```python
from build123d import *

# Parameters (mm, degrees)
F2_R      = 1.5
F3_DEPTH  = 5
F5_D      = 5.25
F5_DEPTH  = 7
F5_TIP    = 1.5772591249
F7_R      = 5
F8_DEPTH  = 2
F10_D     = 5.25
F10_DEPTH = 6.25
F10_TIP   = 1.5772591249
F12_R     = 5
F13_DEPTH = 2
F15_D     = 5.25
F15_DEPTH = 6.25
F15_TIP   = 1.5772591249
F16_R     = 12.5
F17_DEPTH = 9.5
F18_SIZE  = 2.5
F20_DEPTH = 17


with BuildPart() as f1:
    # F0 (on Front) → F1 (revolve)
    with BuildSketch(Plane.XZ):
        Polygon((0, 0), (0, 5), (0, 15.5), (-18, 15.5), (-18, 7), (-20, 7), (-20, 5), (-20, 0), align=None)
    revolve(axis=Axis((-5.3004380733, 0, 0), (-1, 0, 0)))

    # F2 (on face) → F3 (cut)
    with BuildSketch(Plane(origin=(-18, 0, 0), x_dir=(0, -1, 0), z_dir=(-1, 0, 0))):
        with Locations((8.25, 8.25)):
            Circle(F2_R)
        with Locations((-8.25, 8.25)):
            Circle(F2_R)
        with Locations((-8.25, -8.25)):
            Circle(F2_R)
        with Locations((8.25, -8.25)):
            Circle(F2_R)
    extrude(amount=-F3_DEPTH, mode=Mode.SUBTRACT)

    # F5
    with Locations(Plane(origin=(-18, 0, 0), x_dir=(0, -1, 0), z_dir=(-1, 0, 0))):
        with Locations((-8.25, 8.25), (8.25, 8.25), (-8.25, -8.25), (8.25, -8.25)):
            Hole(F5_D / 2, depth=F5_DEPTH)
            with Locations((0, 0, -(F5_DEPTH + F5_TIP / 2))):  # 118° drill point
                Cone(0, F5_D / 2, F5_TIP, mode=Mode.SUBTRACT)

    # F7 (on offset) → F8 (cut)
    with BuildSketch(Plane.XZ.offset(15.5)):
        with Locations((-7, 0)):
            Circle(F7_R)
    extrude(amount=-F8_DEPTH, mode=Mode.SUBTRACT)

    # F10
    with Locations(Plane.XZ.offset(13.5)):
        with Locations((-7, 0)):
            Hole(F10_D / 2, depth=F10_DEPTH)
            with Locations((0, 0, -(F10_DEPTH + F10_TIP / 2))):  # 118° drill point
                Cone(0, F10_D / 2, F10_TIP, mode=Mode.SUBTRACT)

    # F12 (on offset) → F13 (cut)
    with BuildSketch(Plane.XZ.offset(-15.5)):
        with Locations((-8, 0)):
            Circle(F12_R)
    extrude(amount=F13_DEPTH, mode=Mode.SUBTRACT)

    # F15
    with Locations(Plane(origin=(0, 13.5, 0), x_dir=(-1, 0, 0), z_dir=(0, 1, 0))):
        with Locations((8, 0)):
            Hole(F15_D / 2, depth=F15_DEPTH)
            with Locations((0, 0, -(F15_DEPTH + F15_TIP / 2))):  # 118° drill point
                Cone(0, F15_D / 2, F15_TIP, mode=Mode.SUBTRACT)

    # F16 (on face) → F17 (join)
    with BuildSketch(Plane.YZ):
        Circle(F16_R)
    extrude(amount=F17_DEPTH)

    # F18
    f18_edges = [f1.edges().sort_by_distance(p)[0] for p in [
        (9.5, -12.5, 0),
    ]]
    chamfer(f18_edges, length=F18_SIZE)

    # F19 (on face) → F20 (cut)
    with BuildSketch(Plane(origin=(-18, 0, 0), x_dir=(0, -1, 0), z_dir=(-1, 0, 0))):
        with BuildLine():
            Line((-14.6714007511, -5), (-14.6714007511, 5))
            ThreePointArc((-14.6714007511, 5), (-15.5, 0), (-14.6714007511, -5))
        make_face()
        with BuildLine():
            ThreePointArc((14.6714007511, -5), (15.5, 0), (14.6714007511, 5))
            Line((14.6714007511, 5), (14.6714007511, -5))
        make_face()
    extrude(amount=-F20_DEPTH, mode=Mode.SUBTRACT)


solid = f1.part
```
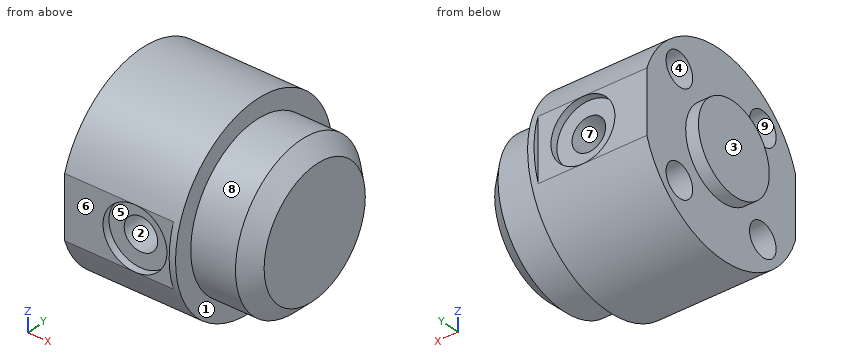
For this review, take the finished solid that the model builds, in its own axes (mm). Face numbers are marked on the shaded views. A direction names the side the tool comes from. Round coordinates to 2 decimals unless told otherwise and drop trailing zeros. Write each loop counter-clockwise with the first axis right and the second up, starting at its lowest first coordinate (ties: lowest second). Pieces come first, ordered by that corner, then holes. Notation, with made-up numbers: (-13, -36) -> (23, -36) arc R20 cw to (23, -21) -> close; hole circle Ø8 at (40, 2). An arc over 180 degrees is marked (long way). One line per question, with ' | ' between items. Start each with the question number.
1) Add section B-B (y = -13). Write out the cut boundary in (x, z) (3 decimals), and give its area (3 significant figures).
2) Wall thickness on line 1 along X through (y, z) = (14.4, 0); line 2 along Z through (x, y) = (-15.5, 8.25) (3 decimals): over which ranges is each line inside the solid? List them lowest first.
3) Machinability: for the marked faces 5, 6, 7, 8 and 9, which of the approach directions +Z, -Z, +X, -X, +Y, -Y give a long, thin tool a straight path to every point of the face, cutting with its end or side? Answer none if there is none.
4) Add section A-A (x = -15.75). Write out the cut boundary in (y, z) (3 decimals), and give its area (3 significant figures).
5) For pin 1 Ø6 at (y, z) = (8.25, 8.25) entering from -X; pin 2 Ø7 at (x, z) = (-7, 0) entering from +Y; pin 3 Ø1.5 at (x, z) = (-8.5, -7) entering from -Y; pin 4 Ø8 at (y, z) = (-4.5, 11.5) entering from +X, all flat-tipped, find the tip position at first contact; note any pin that passes through.
6) Mouldability with a two-part tool opening along X and no side actions: class the marked faces 1, 2, 3 and 4 as +X half, -X half, draft (parallel to the pull), parting line (faces both ways), or undercut.
Reported:
1) outline: (-18, -8.441) -> (0, -8.441) -> (0, 8.441) -> (-18, 8.441) -> close; hole circle Ø5.25 at (-7, 0) | area: 282 mm²
2) line 1: x = -18 to -13, -3 to 0 | line 2: z = -13.122 to -10.875, -5.625 to 5.625, 10.875 to 13.122
3) face 5: -Y | face 6: +Z, -Z, -X, -Y | face 7: +Y | face 8: +X | face 9: -X
4) outline: (-14.671, -5) arc R15.5 ccw to (14.671, -5) -> (14.671, 5) arc R15.5 ccw to (-14.671, 5) -> close; hole circle Ø5.25 at (-8.25, -8.25); hole circle Ø5.25 at (-8.25, 8.25); hole circle Ø5.25 at (8.25, -8.25); hole circle Ø5.25 at (8.25, 8.25) | area: 657 mm²
5) pin 1: stops at x = -18 | pin 2: stops at y = 13.5 | pin 3: stops at y = -14.18 | pin 4: stops at x = 9.5
6) face 1: +X half | face 2: undercut | face 3: -X half | face 4: draft
